from build123d import *

# Parameters (mm, degrees)
SKETCH1_W           = 47.5
SKETCH1_H           = 73
BOSS_EXTRUDE2_DEPTH = 8
CUT_EXTRUDE7_DEPTH  = 6
SKETCH1_9_R         = 2
CUT_EXTRUDE10_DEPTH = 125.324529963


with BuildPart() as part:
    # Sketch1 → Boss-Extrude2 (new body)
    with BuildSketch(Plane(origin=(0, 0, 0), x_dir=(1, 0, 0), z_dir=(0, 1, 0))):
        with Locations((-94.251130157, 1.818690378)):
            Rectangle(SKETCH1_W, SKETCH1_H)
    extrude(amount=BOSS_EXTRUDE2_DEPTH)

    # Sketch1_8 → Cut-Extrude7 (cut)
    with BuildSketch(Plane(origin=(0, 0, 0), x_dir=(1, 0, 0), z_dir=(0, 1, 0))):
        Polygon((-94.251130157, -34.681309622), (-94.251130157, 1.818690378), (-114.001130157, 1.818690378), (-114.001130157, -26.681309622), (-110.001130157, -26.681309622), (-110.001130157, -34.681309622), align=None)
        Polygon((-78.501130157, 38.318690378), (-94.251130157, 38.318690378), (-94.251130157, 1.818690378), (-74.501130157, 1.818690378), (-74.501130157, 30.318690378), (-78.501130157, 30.318690378), align=None)
        Polygon((-94.251130157, 38.318690378), (-110.001130157, 38.318690378), (-110.001130157, 30.318690378), (-114.001130157, 30.318690378), (-114.001130157, 1.818690378), (-94.251130157, 1.818690378), align=None)
        Polygon((-74.501130157, 1.818690378), (-94.251130157, 1.818690378), (-94.251130157, -34.681309622), (-78.501130157, -34.681309622), (-78.501130157, -26.681309622), (-74.501130157, -26.681309622), align=None)
    extrude(amount=CUT_EXTRUDE7_DEPTH, mode=Mode.SUBTRACT)

    # Sketch1_9 → Cut-Extrude10 (cut, through all)
    with BuildSketch(Plane(origin=(0, 0, 0), x_dir=(1, 0, 0), z_dir=(0, 1, 0))):
        with Locations(Location((-114.001130157, 34.318690378, 0), (0, 0, 270))):
            Circle(SKETCH1_9_R)
        with Locations(Location((-74.501130157, 34.318690378, 0), (0, 0, 90))):
            Circle(SKETCH1_9_R)
        with Locations(Location((-114.001130157, -30.681309622, 0), (0, 0, 90))):
            Circle(SKETCH1_9_R)
        with Locations(Location((-74.501130157, -30.681309622, 0), (0, 0, 270))):
            Circle(SKETCH1_9_R)
    extrude(amount=CUT_EXTRUDE10_DEPTH, mode=Mode.SUBTRACT)


solid = part.part
Input: part model. Units: mm. Frame: model coordinates. A direction names the side the tool comes from. Round coordinates to 2 decimals unless told otherwise and drop trailing zeros. Loops run counter-clockwise (first coordinate to the right, second up) from the corner with the lowest first, then second, coordinate; pieces in that order, holes last. Notation, with made-up numbers: (71, 30) -> (121, 30) arc R27 cw to (121, 56) -> close; hole circle Ø11 at (57.25, -14). An arc over 180 degrees is marked (long way). Answer as a JSON object with one key per item and string values. Group by question number.
1) Draft query along X for faces 1 (the flat face through (-76, 3, -30.319)), 2 (the flat face through (-118.001, 4, -1)), 3 (the flat face through (-95, 8, -2)). Return one class per face: +X half, -X half, draft (parallel to the pull), parting line (faces both ways), or undercut.
2) Section query B-B on z = 30. Output: boundary loops of the cut face in (x, y).
3) Section query C-C on z = -5. Output: boundary loops of the cut face in (x, y).
4) Section query D-D on x = -85. Output: boundary loops of the cut face in (y, z).
5) Reachability of faces 4 (the cylindrical face through (-115.35, 3.94, 32.16)), 5 (the flat face through (-78.501, 3, 31)), 6 (the flat face through (-77, 3, 26.681)) from +Z, -Z, +X, -X, +Y, -Y: full face, straight path, thin tool, end or side. Return the list, or none.
6) Section query A-A on y = 1. Output: boundary loops of the cut face in (x, z), plus the area to 3 significant figures.
7) Ray query, L1, parallel to X at y = 1.5, z = 20; L2, parallel to Z at x = -76, y = 5; L3, parallel to Z at x = -113, y = 5.5. Return the intervals inside material, ascending.
8) Pin query (flat end, axial travel): pin 1 (12 mm diameter, centred on x = -96.5, z = -19, fed in from -Y). Return the tip coordinate at first contact, or that it passes through.
Reply:
{
 "1": {"face 1": "undercut", "face 2": "-X half", "face 3": "draft"},
 "2": {"outline": "(-118, 0) -> (-115.88, 0) -> (-115.88, 8) -> (-118, 8) -> close; (-112.12, 0) -> (-110, 0) -> (-110, 6) -> (-78.5, 6) -> (-78.5, 0) -> (-76.38, 0) -> (-76.38, 8) -> (-112.12, 8) -> close; (-72.62, 0) -> (-70.5, 0) -> (-70.5, 8) -> (-72.62, 8) -> close"},
 "3": {"outline": "(-118, 0) -> (-114, 0) -> (-114, 6) -> (-74.5, 6) -> (-74.5, 0) -> (-70.5, 0) -> (-70.5, 8) -> (-118, 8) -> close"},
 "4": {"outline": "(6, -38.32) -> (8, -38.32) -> (8, 34.68) -> (6, 34.68) -> close"},
 "5": {"face 4": "+Y, -Y", "face 5": "+Z, -Z, -Y", "face 6": "-Y"},
 "6": {"outline": "(-118, -38.32) -> (-110, -38.32) -> (-110, -30.32) -> (-114, -30.32) -> (-114, 26.68) -> (-110, 26.68) -> (-110, 34.68) -> (-118, 34.68) -> close; (-78.5, -38.32) -> (-70.5, -38.32) -> (-70.5, 34.68) -> (-78.5, 34.68) -> (-78.5, 26.68) -> (-74.5, 26.68) -> (-74.5, -30.32) -> (-78.5, -30.32) -> close; hole circle Ø4 at (-114, -34.32); hole circle Ø4 at (-114, 30.68); hole circle Ø4 at (-74.5, -34.32); hole circle Ø4 at (-74.5, 30.68)", "area": "662 mm2"},
 "7": {"L1": "x = -118 to -114, -74.5 to -70.5", "L2": "z = -38.32 to -35.64, -32.99 to -30.32, 26.68 to 29.36, 32.01 to 34.68", "L3": "z = -38.32 to -36.05, -32.59 to -30.32, 26.68 to 28.95, 32.41 to 34.68"},
 "8": {"pin 1": "stops at y = 6"}
}
